Could you check a few things on this model? Use its own coordinates, in mm. Round coordinates to 2 decimals unless told otherwise and drop trailing zeros. Loops run counter-clockwise (first coordinate to the right, second up) from the corner with the lowest first, then second, coordinate; pieces in that order, holes last. Notation, with made-up numbers: (43.25, 51.5) -> (98.25, 51.5) arc R28 ccw to (98.25, 75.5) -> close; hole circle Ø11 at (43, 25). An arc over 180 degrees is marked (long way). Write each question's results on one line, items separated by ' | '. Start each with the question number.
1) Imagine slicing it at A-A, the plane y = -63.5. List the corners of the cut face in (x, z) for me (3 decimals), plus the area to 3 significant figures.
2) If I drill on probe 1 along Y at (x, z) = (8, -95.25) (3 decimals); probe 2 along Z at (x, y) = (3, 82) (3 decimals); probe 3 along Y at (x, z) = (8.25, 25.5), over which ranges is the centre line in solid material (lowest first)?
3) Imagine slicing it at B-B, the plane x = 9.25. Give the number of separate pieces and of enclosed holes in the cut face, plus the area to 3 significant figures.
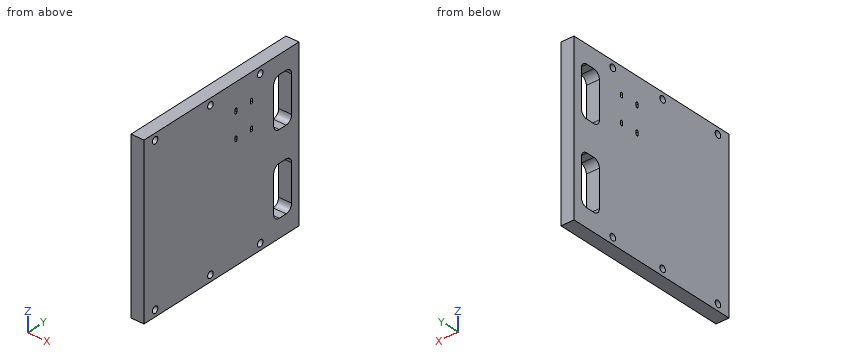
from build123d import *

# Parameters (mm, degrees)
SKETCH1_W           = 161.925
SKETCH1_H           = 177.8
SKETCH1_R           = 3.175
BOSS_EXTRUDE1_DEPTH = 12.7


with BuildPart() as part:
    # Sketch1 → Boss-Extrude1 (new body)
    with BuildSketch(Plane(origin=(0, 0, 0), x_dir=(0, 0, -1), z_dir=(1, 0, 0))):
        with Locations((20.6375, 12.7)):
            Rectangle(SKETCH1_W, SKETCH1_H)
        with Locations((-53.975, -63.5)):
            Circle(SKETCH1_R, mode=Mode.SUBTRACT)
        with Locations((-53.975, 0)):
            Circle(SKETCH1_R, mode=Mode.SUBTRACT)
        with Locations((95.25, -63.5)):
            Circle(SKETCH1_R, mode=Mode.SUBTRACT)
        with Locations((95.25, 0)):
            Circle(SKETCH1_R, mode=Mode.SUBTRACT)
        with BuildLine():
            ThreePointArc((-33.455, 30.43), (-32.255, 29.23), (-33.455, 28.03))
            Line((-33.455, 28.03), (-36.055, 28.03))
            ThreePointArc((-36.055, 28.03), (-37.255, 29.23), (-36.055, 30.43))
            Line((-36.055, 30.43), (-33.455, 30.43))
        make_face(mode=Mode.SUBTRACT)
        with BuildLine():
            Line((-36.055, 48.17), (-33.455, 48.17))
            ThreePointArc((-33.455, 48.17), (-32.255, 46.97), (-33.455, 45.77))
            Line((-33.455, 45.77), (-36.055, 45.77))
            ThreePointArc((-36.055, 45.77), (-37.255, 46.97), (-36.055, 48.17))
        make_face(mode=Mode.SUBTRACT)
        with BuildLine():
            ThreePointArc((-8.915, 30.43), (-7.715, 29.23), (-8.915, 28.03))
            Line((-8.915, 28.03), (-11.515, 28.03))
            ThreePointArc((-11.515, 28.03), (-12.715, 29.23), (-11.515, 30.43))
            Line((-11.515, 30.43), (-8.915, 30.43))
        make_face(mode=Mode.SUBTRACT)
        with Locations((-53.975, 57.15)):
            Circle(SKETCH1_R, mode=Mode.SUBTRACT)
        with BuildLine():
            Line((-42.588896299, 78.866901715), (-42.588896299, 86.823202123))
            ThreePointArc((-42.588896299, 86.823202123), (-40.729024359, 91.313330183), (-36.238896299, 93.173202123))
            Line((-36.238896299, 93.173202123), (-0.602666303, 93.173202123))
            ThreePointArc((-0.602666303, 93.173202123), (3.887461758, 91.313330183), (5.747333697, 86.823202123))
            Line((5.747333697, 86.823202123), (5.747333697, 78.866901715))
            ThreePointArc((5.747333697, 78.866901715), (3.887461758, 74.376773654), (-0.602666303, 72.516901715))
            Line((-0.602666303, 72.516901715), (-36.238896299, 72.516901715))
            ThreePointArc((-36.238896299, 72.516901715), (-40.729024359, 74.376773654), (-42.588896299, 78.866901715))
        make_face(mode=Mode.SUBTRACT)
        with Locations((95.25, 57.15)):
            Circle(SKETCH1_R, mode=Mode.SUBTRACT)
        with BuildLine():
            ThreePointArc((41.877666303, 72.516901715), (37.387538242, 74.376773654), (35.527666303, 78.866901715))
            Line((35.527666303, 78.866901715), (35.527666303, 86.823202123))
            ThreePointArc((35.527666303, 86.823202123), (37.387538242, 91.313330183), (41.877666303, 93.173202123))
            Line((41.877666303, 93.173202123), (77.513896299, 93.173202123))
            ThreePointArc((77.513896299, 93.173202123), (82.004024359, 91.313330183), (83.863896299, 86.823202123))
            Line((83.863896299, 86.823202123), (83.863896299, 78.866901715))
            ThreePointArc((83.863896299, 78.866901715), (82.004024359, 74.376773654), (77.513896299, 72.516901715))
            Line((77.513896299, 72.516901715), (41.877666303, 72.516901715))
        make_face(mode=Mode.SUBTRACT)
        with BuildLine():
            ThreePointArc((-11.515, 45.77), (-12.715, 46.97), (-11.515, 48.17))
            Line((-11.515, 48.17), (-8.915, 48.17))
            ThreePointArc((-8.915, 48.17), (-7.715, 46.97), (-8.915, 45.77))
            Line((-8.915, 45.77), (-11.515, 45.77))
        make_face(mode=Mode.SUBTRACT)
    extrude(amount=BOSS_EXTRUDE1_DEPTH)


solid = part.part
Checked values:
1) outline: (0, -101.6) -> (12.7, -101.6) -> (12.7, -98.425) -> (0, -98.425) -> close; (0, -92.075) -> (12.7, -92.075) -> (12.7, 50.8) -> (0, 50.8) -> close; (0, 57.15) -> (12.7, 57.15) -> (12.7, 60.325) -> (0, 60.325) -> close | area: 1,900 mm^2
2) probe 1: -76.2 to -66.675, -60.325 to -3.175, 3.175 to 53.975, 60.325 to 101.6 | probe 2: -101.6 to -83.864, -35.528 to -5.747, 42.589 to 60.325 | probe 3: -76.2 to 72.52, 93.17 to 101.6
3) separate pieces: 1 | enclosed holes: 12 | area: 26,600 mm^2
